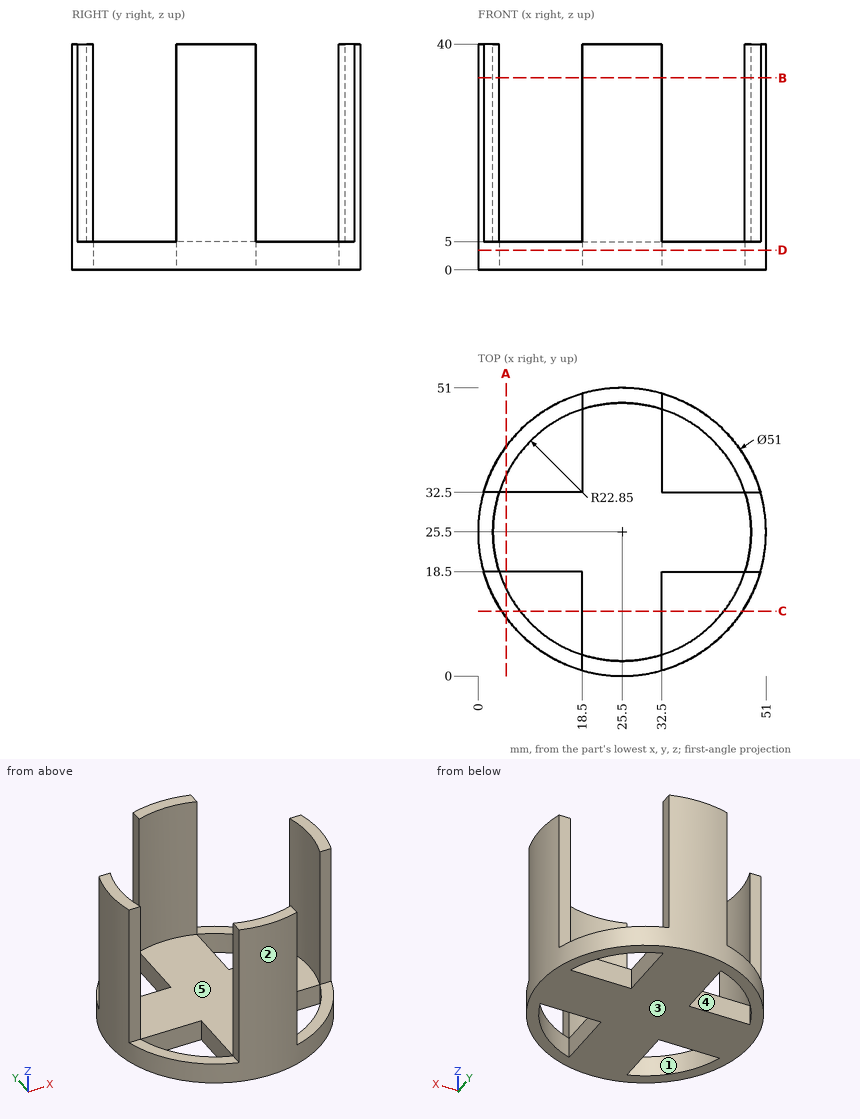
Verification items for this drawing (mm, ordinates from the low corner). A direction names the side the tool comes from. Round coordinates to 2 decimals unless told otherwise and drop trailing zeros. Loops run counter-clockwise (first coordinate to the right, second up) from the corner with the lowest first, then second, coordinate; pieces in that order, holes last. Notation, with made-up numbers: (70, 37) -> (91, 37) arc R23 cw to (91, 69) -> close; hole circle Ø5 at (29.25, -11). An arc over 180 degrees is marked (long way). Write item = value, one per line. Start each with the question number.
1) Gauge pin test, flat ends, axial feed: pin 1 Ø5.5 at (x, y) = (43, 41.5) entering from +Z; pin 2 Ø5.5 at (x, z) = (13.5, 2.5) entering from -Y; pin 3 Ø2.5 at (x, z) = (11, 2) entering from +Y. Record the tip position at first contact, or that the pin passes through.
2) Sectioned sample at C-C, the plane y = 11.5. Record the cut outline in (x, z).
3) Set-up check for the marked faces 4 and 5: record each of +Z, -Z, +X, -X, +Y, -Y from which the full face is reachable in a straight line by a thin tool's end or side.
4) Sectioned sample at A-A, the plane x = 5. Record the cut outline in (y, z), plus the area to 3 significant figures.
5) Release check for a two-part mould opening along X. For the marked faces 1, 2 and 3 record: released by +X, released by -X, zero draft, split by the parting line, or undercut.
6) Sectioned sample at B-B, the plane z = 34. Record the cut outline in (x, y), plus the area to 3 significant figures.
7) Thickness scan on probe 1 along Z at (x, y) = (14, 22); probe 2 along X at (y, z) = (22, 35); probe 3 along X at (y, z) = (30.5, 11) (3 decimals). Record the ranges inside material, lowest first.
8) Sectioned sample at D-D, the plane z = 3.5. Record the cut outline in (x, y).
Results are:
q1.pin_1 = 5
q1.pin_2 = 1.74
q1.pin_3 = 47.29
q2.outline = (4.19, 0) -> (7.44, 0) -> (7.44, 5) -> (4.19, 5) -> close; (18.5, 0) -> (32.5, 0) -> (32.5, 5) -> (18.5, 5) -> close; (43.56, 0) -> (46.81, 0) -> (46.81, 5) -> (43.56, 5) -> close
q3.face_4 = +Z, -Z
q3.face_5 = +Z
q4.outline = (10.33, 0) -> (15.41, 0) -> (15.41, 5) -> (10.33, 5) -> close; (18.5, 0) -> (32.5, 0) -> (32.5, 5) -> (18.5, 5) -> close; (35.59, 0) -> (40.67, 0) -> (40.67, 5) -> (35.59, 5) -> close
q4.area = 121 mm^2
q5.face_1 = undercut
q5.face_2 = split by the parting line
q5.face_3 = zero draft
q6.outline = (0.98, 18.5) -> (3.75, 18.5) arc R22.85 cw to (3.75, 32.5) -> (0.98, 32.5) arc R25.5 ccw to start; (18.5, 0.98) arc R25.5 ccw to (32.5, 0.98) -> (32.5, 3.75) arc R22.85 cw to (18.5, 3.75) -> close; (18.5, 47.25) arc R22.85 cw to (32.5, 47.25) -> (32.5, 50.02) arc R25.5 ccw to (18.5, 50.02) -> close; (47.25, 18.5) -> (50.02, 18.5) arc R25.5 ccw to (50.02, 32.5) -> (47.25, 32.5) arc R22.85 cw to start
q6.area = 151 mm^2
q7.probe_1 = 0 to 5
q7.probe_2 = 0.24 to 2.92, 48.08 to 50.76
q7.probe_3 = 0.495 to 3.204, 47.796 to 50.505
q8.outline = circle Ø51 at (25.5, 25.5); hole (3.75, 18.5) arc R22.85 ccw to (18.5, 3.75) -> (18.5, 18.5) -> close; hole (3.75, 32.5) -> (18.5, 32.5) -> (18.5, 47.25) arc R22.85 ccw to start; hole (32.5, 3.75) arc R22.85 ccw to (47.25, 18.5) -> (32.5, 18.5) -> close; hole (32.5, 32.5) -> (47.25, 32.5) arc R22.85 ccw to (32.5, 47.25) -> close
